The listing builds one solid part. Answer for the finished solid, in the listing's coordinates (mm). Face numbers are marked on the shaded views. A direction names the side the tool comes from. Give positions to 0.01 mm unless a question says otherwise; leave off trailing zeros. Write each loop counter-clockwise with the first axis right and the second up, starting at its lowest first coordinate (ties: lowest second). Pieces come first, ordered by that corner, then holes. Notation, with made-up numbers: (4.5, 12) - (17.5, 12) arc R11 cw to (17.5, 30) - close; hole circle Ø2 at (30.5, 7.5). An arc over 180 degrees is marked (long way). Use a Markdown table: item, result. Add a question column.
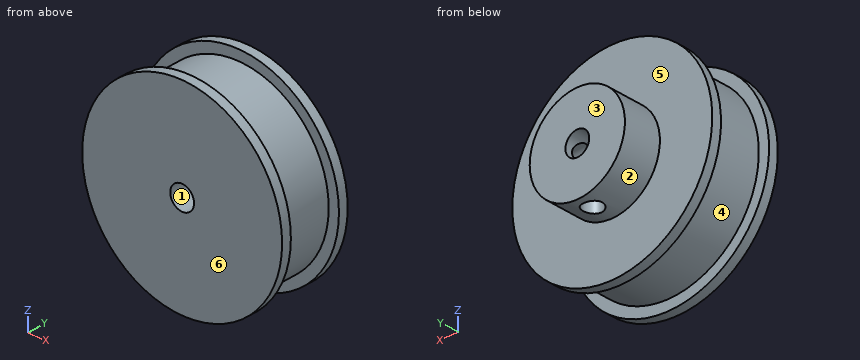
from build123d import *

# Parameters (mm, degrees)
SKETCH1_R           = 21
BOSS_EXTRUDE1_DEPTH = 2
SKETCH2_R           = 18.85
BOSS_EXTRUDE2_DEPTH = 11
SKETCH3_R           = 21
BOSS_EXTRUDE3_DEPTH = 2
SKETCH4_R           = 10
BOSS_EXTRUDE4_DEPTH = 8
SKETCH5_R           = 2.5
CUT_EXTRUDE1_DEPTH  = 24
SKETCH6_R           = 2
CUT_EXTRUDE2_DEPTH  = 22
CIRPATTERN1_COUNT   = 2
CIRPATTERN1_ANGLE   = 90


with BuildPart() as part:
    # Sketch1 → Boss-Extrude1 (new body)
    with BuildSketch(Plane(origin=(0, 0, 0), x_dir=(1, 0, 0), z_dir=(0, 1, 0))):
        Circle(SKETCH1_R)
    extrude(amount=BOSS_EXTRUDE1_DEPTH)

    # Sketch2 → Boss-Extrude2 (add)
    with BuildSketch(Plane(origin=(0, 2, 0), x_dir=(1, 0, 0), z_dir=(0, 1, 0))):
        Circle(SKETCH2_R)
    extrude(amount=BOSS_EXTRUDE2_DEPTH)

    # Sketch3 → Boss-Extrude3 (add)
    with BuildSketch(Plane(origin=(0, 13, 0), x_dir=(1, 0, 0), z_dir=(0, 1, 0))):
        Circle(SKETCH3_R)
    extrude(amount=BOSS_EXTRUDE3_DEPTH)

    # Sketch4 → Boss-Extrude4 (add)
    with BuildSketch(Plane(origin=(0, 15, 0), x_dir=(1, 0, 0), z_dir=(0, 1, 0))):
        Circle(SKETCH4_R)
    extrude(amount=BOSS_EXTRUDE4_DEPTH)

    # Sketch5 → Cut-Extrude1 (cut, through all)
    with BuildSketch(Plane(origin=(0, 23, 0), x_dir=(1, 0, 0), z_dir=(0, 1, 0))):
        Circle(SKETCH5_R)
    extrude(amount=-CUT_EXTRUDE1_DEPTH, mode=Mode.SUBTRACT)

    # Sketch6 → Cut-Extrude2 (cut, through all)
    with BuildSketch(Plane.XY):
        with Locations((0, 19.5)):
            Circle(SKETCH6_R)
    cut_extrude2 = extrude(amount=-CUT_EXTRUDE2_DEPTH, mode=Mode.SUBTRACT)

    # CirPattern1: Cut-Extrude2 ×2 about axis
    cirpattern1_axis = Axis((0, 23, 0), (0, -1, 0))
    for i in range(1, CIRPATTERN1_COUNT):
        add(cut_extrude2.rotate(cirpattern1_axis, i * CIRPATTERN1_ANGLE / (CIRPATTERN1_COUNT - 1)), mode=Mode.SUBTRACT)


solid = part.part
1. The part is cut by section A-A (z = 0). Give the vertices of the cut face in (x, y), and give its area (3 significant figures).
2. Consider L1, parallel to Y at x = -11.5, z = 17; L2, parallel to Y at x = 3, z = 0; L3, parallel to Y at x = -12, z = -4. Determine where each line is inside the solid, lowest interval first. Write a range as [from, to].
3. Which of the six approach directions +Z, -Z, +X, -X, +Y, -Y give full straight-line access (tool end or side, diameter ignored) to the marked faces 4, 5 and 6?
4. Given P1, Ø4, axis at y = 5.5, z = 0.5, coming from the -X side; P2, Ø5, axis at x = -5, y = 8.5, coming from the +Z side; P3, Ø10, axis at x = -6.5, y = 11.5, coming from the +Z side, each flat-ended and moving along its own axis, determine where each tip first touches the part or whether it passes through.
5. For a pull along Z with two mould halves and no side action, classify the marked faces 1, 2 and 3 as released by +Z, released by -Z, zero draft, split by the parting line, or undercut.
6. The part is cut by section B-B (x = 0). Give the vertices of the cut face in (y, z), and give its area (3 significant figures).
7. The part is cut by section D-D (y = 16). Give the vertices of the cut face in (x, z), and give its area (3 significant figures).
8. The part is cut by section C-C (y = 19.5). Give the vertices of the cut face in (x, z), and give its area (3 significant figures).
Check values:
| question | item | result |
|---|---|---|
| 1 | outline | (-21, 0) - (-2.5, 0) - (-2.5, 23) - (-10, 23) - (-10, 15) - (-21, 15) - (-21, 13) - (-18.85, 13) - (-18.85, 2) - (-21, 2) - close; (2.5, 0) - (21, 0) - (21, 2) - (18.85, 2) - (18.85, 13) - (21, 13) - (21, 15) - (10, 15) - (10, 17.5) - (2.5, 17.5) - close; (2.5, 21.5) - (10, 21.5) - (10, 23) - (2.5, 23) - close |
| 1 | area | 598 mm2 |
| 2 | L1 | y = [0, 2], [13, 15] |
| 2 | L2 | y = [0, 17.5], [21.5, 23] |
| 2 | L3 | y = [0, 15] |
| 3 | face 4 | none |
| 3 | face 5 | +Y |
| 3 | face 6 | +Z, -Z, +X, -X, -Y |
| 4 | P1 | stops at x = -18.85 |
| 4 | P2 | stops at z = 18.68 |
| 4 | P3 | stops at z = 20.93 |
| 5 | face 1 | undercut |
| 5 | face 2 | split by the parting line |
| 5 | face 3 | zero draft |
| 6 | outline | (0, -21) - (2, -21) - (2, -18.85) - (13, -18.85) - (13, -21) - (15, -21) - (15, -10) - (17.5, -10) - (17.5, -2.5) - (0, -2.5) - close; (0, 2.5) - (23, 2.5) - (23, 10) - (15, 10) - (15, 21) - (13, 21) - (13, 18.85) - (2, 18.85) - (2, 21) - (0, 21) - close; (21.5, -10) - (23, -10) - (23, -2.5) - (21.5, -2.5) - close |
| 6 | area | 598 mm2 |
| 7 | outline | circle Ø20 at (0, 0); hole circle Ø5 at (0, 0) |
| 7 | area | 295 mm2 |
| 8 | outline | (-2, -9.8) - (-2, -1.5) arc R2.5 cw to (1.5, 2) - (9.8, 2) arc R10 ccw (long way) to start; (2, -9.8) arc R10 ccw to (9.8, -2) - (2, -2) - close |
| 8 | area | 233 mm2 |
